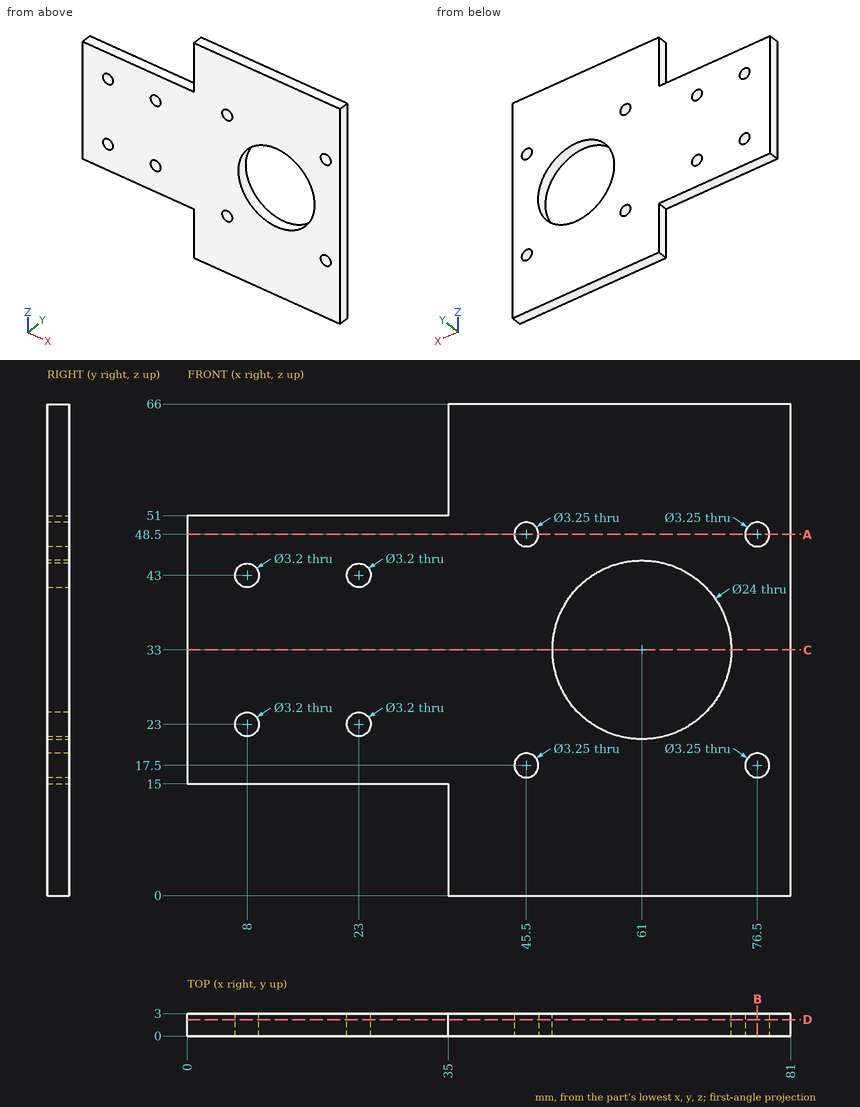
Geometry: see drawing. Coordinates: mm, zero at the bounding-box minimum. Give positions to 0.01 mm unless a question says otherwise; leave off trailing zeros. Write each loop counter-clockwise with the first axis right and the second up, starting at its lowest first coordinate (ties: lowest second). Pieces come first, ordered by that corner, then holes. Notation, with made-up numbers: M 73,50.5 L 117,50.5 A30 ccw 117,79.5 Z; hole C 20.25,-27 d2. An arc over 180 degrees is marked long. Answer as a JSON object with one key per item and string values.
Q1. Ray query, line 1 along Z through (x, y) = (76.5, 1.2) (3 decimals); line 2 along X through (y, z) = (1.9, 48.5) (3 decimals); line 3 along X through (y, z) = (2.25, 43). Return the intervals inside material, ascending.
Geometry check:
{"line 1": "z = 0 to 15.875, 19.125 to 46.875, 50.125 to 66", "line 2": "x = 0 to 43.875, 47.125 to 74.875, 78.125 to 81", "line 3": "x = 0 to 6.4, 9.6 to 21.4, 24.6 to 54.37, 67.63 to 81"}
Q2. Contact query for flat-ended pins moving along their axis: P1, Ø1.5, axis at y = 1, z = 60, coming from the -X side; P2, Ø1.5, axis at x = 13.5, y = 2, coming from the +Z side. Output: stop coordinate, or through.
Geometry check:
{"P1": "stops at x = 35", "P2": "stops at z = 51"}
Q3. Cut plane B-B, the plane x = 76.5. Return the cut outline in (y, z) (3 decimals).
Geometry check:
{"outline": "M 0,0 L 3,0 L 3,15.875 L 0,15.875 Z; M 0,19.125 L 3,19.125 L 3,46.875 L 0,46.875 Z; M 0,50.125 L 3,50.125 L 3,66 L 0,66 Z"}
Q4. Cut plane D-D, the plane y = 2.2. Count the separate pieces of the cut face and the enclosed holes in it, then the cut area to 3 significant figures.
Geometry check:
{"separate pieces": "1", "enclosed holes": "9", "area": "3,780 mm^2"}
Q5. Cut plane C-C, the plane z = 33. Return the cut outline in (x, y), then the cut area to 3 significant figures.
Geometry check:
{"outline": "M 0,0 L 49,0 L 49,3 L 0,3 Z; M 73,0 L 81,0 L 81,3 L 73,3 Z", "area": "171 mm^2"}
Q6. Cut plane A-A, the plane z = 48.5. Return the cut outline in (x, y) (3 decimals), then the cut area to 4 significant figures.
Geometry check:
{"outline": "M 0,0 L 43.875,0 L 43.875,3 L 0,3 Z; M 47.125,0 L 74.875,0 L 74.875,3 L 47.125,3 Z; M 78.125,0 L 81,0 L 81,3 L 78.125,3 Z", "area": "223.5 mm^2"}
